```python
from build123d import *

# Parameters (mm, degrees)
BOSS_EXTRUDE1_DEPTH      = 55
BOSS_EXTRUDE1_DEPTH_BACK = 55
SKETCH4_W                = 6.5
SKETCH4_H                = 5.004744749
BOSS_EXTRUDE3_DEPTH      = 10


with BuildPart() as part:
    # Sketch2 → Boss-Extrude1 (new, two sides: drawn at the far end of the back side and taken through both)
    with BuildSketch(Plane.XY.offset(-BOSS_EXTRUDE1_DEPTH_BACK)):
        with BuildLine():
            Line((25.528440089, 3.245255251), (30.999590193, 3.245255251))
            ThreePointArc((30.999590193, 3.245255251), (31.382758391, 4.08570216), (31.514015141, 5))
            ThreePointArc((31.514015141, 5), (27.349717301, 8.11874325), (25.528440089, 3.245255251))
        make_face()
    extrude(amount=BOSS_EXTRUDE1_DEPTH + BOSS_EXTRUDE1_DEPTH_BACK)

    # Sketch4 → Boss-Extrude3 (add)
    with BuildSketch(Plane.XY.offset(43)):
        with Locations((28.264015141, 5.747627625)):
            Rectangle(SKETCH4_W, SKETCH4_H)
    boss_extrude3 = extrude(amount=-BOSS_EXTRUDE3_DEPTH)

    # Mirror1: Boss-Extrude3 across plane
    add(boss_extrude3.mirror(Plane.XY))


solid = part.part
```
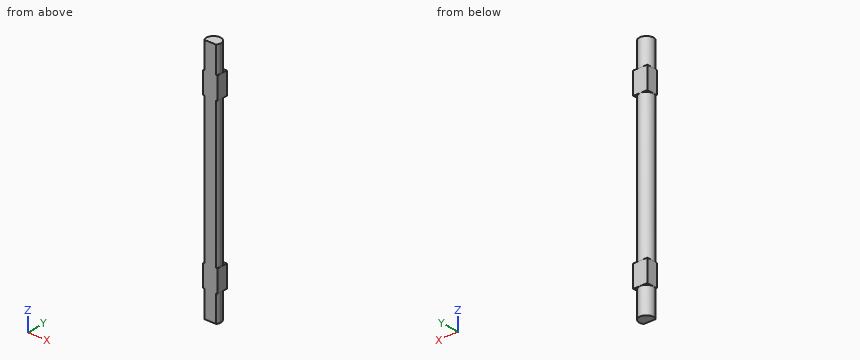
For this review, take the finished solid that the model builds, in its own axes (mm). Give positions to 0.01 mm unless a question says otherwise; leave off trailing zeros. Loops run counter-clockwise (first coordinate to the right, second up) from the corner with the lowest first, then second, coordinate; pieces in that order, holes last. Notation, with made-up numbers: M 17.5,65 L 49.5,65 A6 ccw 49.5,69 Z; hole C 23.5,56.5 d10. An arc over 180 degrees is marked long. One line per item, written item: value. Start each with the question number.
Q1. Add section A-A (x = 29.5). Give the boundary of the cut face in (y, z).
Q2. Add section B-B (y = 6.85). Give the boundary of the cut face in (x, z), and give its area (3 significant figures).
Q3. Clearance check with a flat-ended pin moving along its axis: pin 1 Ø0.6 at (x, y) = (31.5, 4.5) entering from +Z. State where the tip first meets the part, or that it passes through.
Q4. For L1, parallel to X at y = 5.35, z = 22; L2, parallel to Y at x = 30, z = -21.5; L3, parallel to X at y = 7.4, z = -6, list the stretches that pass through material, from the lowest coordinate up.
Q5. Add section C-C (z = -10.5). Give the boundary of the cut face in (x, y).
Reply:
1. outline: M 3.25,-55 L 8.01,-55 L 8.01,-43 L 8.25,-43 L 8.25,-33 L 8.01,-33 L 8.01,33 L 8.25,33 L 8.25,43 L 8.01,43 L 8.01,55 L 3.25,55 Z
2. outline: M 25.01,-43 L 25.59,-43 L 25.59,-55 L 30.94,-55 L 30.94,-43 L 31.51,-43 L 31.51,-33 L 30.94,-33 L 30.94,33 L 31.51,33 L 31.51,43 L 30.94,43 L 30.94,55 L 25.59,55 L 25.59,43 L 25.01,43 L 25.01,33 L 25.59,33 L 25.59,-33 L 25.01,-33 Z
2. area: 611 mm²
3. pin 1: z = 55
4. L1: 25.03 to 31.5
4. L2: 3.25 to 7.75
4. L3: 26.07 to 30.46
5. outline: M 25.53,3.25 L 31,3.25 A3.25 ccw long Z
